Verification items for the finished model (mm, model axes). Face numbers are marked on the shaded views. A direction names the side the tool comes from. Give positions to 0.01 mm unless a question says otherwise; leave off trailing zeros. Order: outer loops, then holes, each group sorted by start corner. A loop starts at its lowest first (then second) coordinate and runs counter-clockwise, first axis right, second up. Notation, with made-up numbers: (1, 13) - (42, 13) arc R11 ccw to (42, 27) - close; hole circle Ø8 at (-17, 14). An arc over 180 degrees is marked (long way). Answer as a JSON object with one key per item and string values. Group by question number.
(1) Thickness scan on line 1 (Y direction, x = 20, z = 18); line 2 (X direction, y = -5, z = -10); line 3 (Z direction, x = -9.5, y = 11). Record the ranges inside material, lowest first.
(2) Section check B-B (x = 1). Record the boundary of the cut face in (y, z).
(3) Section check C-C (z = 12). Record the boundary of the cut face in (x, y), then the cut area to 3 significant figures.
(4) Section check D-D (x = -16.25). Record the boundary of the cut face in (y, z).
(5) Depth check by flat-ended pin: pin 1 Ø6.5 at (x, z) = (16.25, 12) entering from -Y; pin 2 Ø4 at (x, z) = (12.5, -2) entering from +Y; pin 3 Ø1.2 at (x, z) = (15.5, -10.5) entering from -Y; pin 4 Ø1 at (x, z) = (18, 11) entering from +Y. Enter the tip coordinate at first touch or a pass-through.
(6) Section check A-A (y = 17). Record the boundary of the cut face in (x, z).
(7) Access from +Z, -Z, +X, -X, +Y, -Y to the whole of each face (thin tool, end or side, straight path). Record for the marked faces 1, 2 and 3.
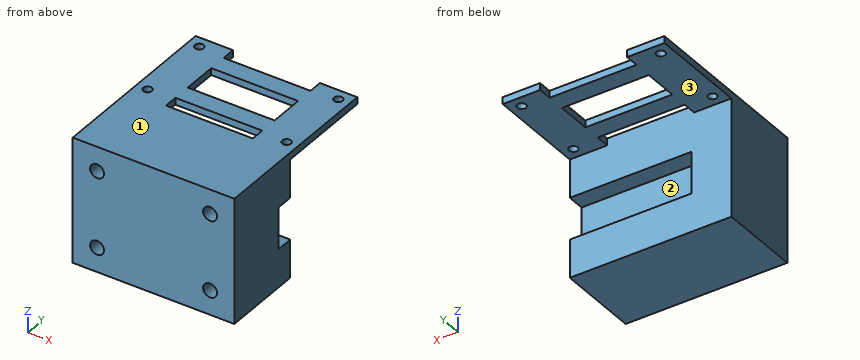
```python
from build123d import *

# Parameters (mm, degrees)
SKETCH1_W           = 46.5
SKETCH1_H           = 34
BOSS_EXTRUDE1_DEPTH = 13.75
SKETCH2_W           = 46.5
SKETCH2_H           = 42.25
BOSS_EXTRUDE2_DEPTH = 2
CUT_EXTRUDE1_REACH  = 62.18
SKETCH3_R           = 1.25
SKETCH3_W           = 25
SKETCH3_H           = 10
SKETCH4_W           = 35
SKETCH4_H           = 12
CUT_EXTRUDE2_DEPTH  = 5
SKETCH6_W           = 46.5
SKETCH6_H           = 36
SKETCH6_R           = 2
BOSS_EXTRUDE3_DEPTH = 10
SKETCH7_W           = 25
SKETCH7_H           = 4
CUT_EXTRUDE3_DEPTH  = 10


with BuildPart() as part:
    # Sketch1 → Boss-Extrude1 (new body)
    with BuildSketch(Plane(origin=(0, 0, 0), x_dir=(1, 0, 0), z_dir=(0, 1, 0))):
        Rectangle(SKETCH1_W, SKETCH1_H)
    extrude(amount=BOSS_EXTRUDE1_DEPTH)

    # Sketch2 → Boss-Extrude2 (add)
    with BuildSketch(Plane.XY.offset(17)):
        with Locations((0, 21.125)):
            Rectangle(SKETCH2_W, SKETCH2_H)
    extrude(amount=BOSS_EXTRUDE2_DEPTH)

    # Sketch3 → Cut-Extrude1 (cut, up to next)
    with BuildSketch(Plane.XY.offset(19), mode=Mode.PRIVATE) as cut_extrude1_sk1:
        with Locations((-20, 39)):
            Circle(SKETCH3_R)
    cut_extrude1_tool1 = extrude(cut_extrude1_sk1.sketch, amount=-CUT_EXTRUDE1_REACH, mode=Mode.PRIVATE) & part.part
    # Sketch3 → Cut-Extrude1 (cut, up to next)
    with BuildSketch(Plane.XY.offset(19), mode=Mode.PRIVATE) as cut_extrude1_sk2:
        with Locations(Location((20, 39, 0), (0, 0, 180))):
            Circle(SKETCH3_R)
    cut_extrude1_tool2 = extrude(cut_extrude1_sk2.sketch, amount=-CUT_EXTRUDE1_REACH, mode=Mode.PRIVATE) & part.part
    # Sketch3 → Cut-Extrude1 (cut, up to next)
    with BuildSketch(Plane.XY.offset(19), mode=Mode.PRIVATE) as cut_extrude1_sk3:
        with Locations((20, 17)):
            Circle(SKETCH3_R)
    cut_extrude1_tool3 = extrude(cut_extrude1_sk3.sketch, amount=-CUT_EXTRUDE1_REACH, mode=Mode.PRIVATE) & part.part
    # Sketch3 → Cut-Extrude1 (cut, up to next)
    with BuildSketch(Plane.XY.offset(19), mode=Mode.PRIVATE) as cut_extrude1_sk4:
        with Locations(Location((-20, 17, 0), (0, 0, 180))):
            Circle(SKETCH3_R)
    cut_extrude1_tool4 = extrude(cut_extrude1_sk4.sketch, amount=-CUT_EXTRUDE1_REACH, mode=Mode.PRIVATE) & part.part
    # Sketch3 → Cut-Extrude1 (cut, up to next)
    with BuildSketch(Plane.XY.offset(19), mode=Mode.PRIVATE) as cut_extrude1_sk5:
        with Locations((0, 28)):
            Rectangle(SKETCH3_W, SKETCH3_H)
    cut_extrude1_tool5 = extrude(cut_extrude1_sk5.sketch, amount=-CUT_EXTRUDE1_REACH, mode=Mode.PRIVATE) & part.part
    add(cut_extrude1_tool1.solids().sort_by_distance((-20, 39, 19))[0], mode=Mode.SUBTRACT)
    add(cut_extrude1_tool2.solids().sort_by_distance((20, 39, 19))[0], mode=Mode.SUBTRACT)
    add(cut_extrude1_tool3.solids().sort_by_distance((20, 17, 19))[0], mode=Mode.SUBTRACT)
    add(cut_extrude1_tool4.solids().sort_by_distance((-20, 17, 19))[0], mode=Mode.SUBTRACT)
    add(cut_extrude1_tool5.solids().sort_by_distance((0, 28, 19))[0], mode=Mode.SUBTRACT)

    # Sketch4 → Cut-Extrude2 (cut)
    with BuildSketch(Plane(origin=(0, 13.75, 0), x_dir=(1, 0, 0), z_dir=(0, 1, 0))):
        with Locations((5.75, 0)):
            Rectangle(SKETCH4_W, SKETCH4_H)
    extrude(amount=-CUT_EXTRUDE2_DEPTH, mode=Mode.SUBTRACT)

    # Sketch6 → Boss-Extrude3 (add)
    with BuildSketch(Plane.XZ):
        with Locations((0, 1)):
            Rectangle(SKETCH6_W, SKETCH6_H)
        with Locations(Location((16.25, -10, 0), (0, 0, 270))):
            Circle(SKETCH6_R, mode=Mode.SUBTRACT)
        with Locations(Location((-16.25, -10, 0), (0, 0, 270))):
            Circle(SKETCH6_R, mode=Mode.SUBTRACT)
        with Locations(Location((-16.25, 12, 0), (0, 0, 270))):
            Circle(SKETCH6_R, mode=Mode.SUBTRACT)
        with Locations(Location((16.25, 12, 0), (0, 0, 270))):
            Circle(SKETCH6_R, mode=Mode.SUBTRACT)
    extrude(amount=BOSS_EXTRUDE3_DEPTH)

    # Sketch7 → Cut-Extrude3 (cut)
    with BuildSketch(Plane(origin=(0, 0, 17), x_dir=(-1, 0, 0), z_dir=(0, 0, -1))):
        with Locations((0, 15.75)):
            Rectangle(SKETCH7_W, SKETCH7_H)
        with Locations((0, 40.25)):
            Rectangle(SKETCH7_W, SKETCH7_H)
    extrude(amount=-CUT_EXTRUDE3_DEPTH, mode=Mode.SUBTRACT)


solid = part.part
```
Solutions:
{
 "1": {"line 1": "y = -10 to 15.75, 18.25 to 37.75, 40.25 to 42.25", "line 2": "x = -23.25 to -18.25, -14.25 to 14.25, 18.25 to 23.25", "line 3": "z = -17 to -6, 6 to 19"},
 "2": {"outline": "(-10, -17) - (13.75, -17) - (13.75, -6) - (8.75, -6) - (8.75, 6) - (13.75, 6) - (13.75, 19) - (-10, 19) - close; (17.75, 17) - (23, 17) - (23, 19) - (17.75, 19) - close; (33, 17) - (38.25, 17) - (38.25, 19) - (33, 19) - close"},
 "3": {"outline": "(-23.25, -10) - (-18.25, -10) - (-18.25, 0) - (-14.25, 0) - (-14.25, -10) - (14.25, -10) - (14.25, 0) - (18.25, 0) - (18.25, -10) - (23.25, -10) - (23.25, 13.75) - (-23.25, 13.75) - close", "area": "1,020 mm2"},
 "4": {"outline": "(-10, -17) - (13.75, -17) - (13.75, 17) - (42.25, 17) - (42.25, 19) - (-10, 19) - (-10, 14) - (0, 14) - (0, 10) - (-10, 10) - (-10, -8) - (0, -8) - (0, -12) - (-10, -12) - close"},
 "5": {"pin 1": "stops at y = -10", "pin 2": "stops at y = 8.75", "pin 3": "stops at y = 0", "pin 4": "stops at y = 13.75"},
 "6": {"outline": "(-23.25, 17) - (-21.25, 17) - (-21.25, 19) - (-23.25, 19) - close; (-18.75, 17) - (-12.5, 17) - (-12.5, 19) - (-18.75, 19) - close; (12.5, 17) - (18.75, 17) - (18.75, 19) - (12.5, 19) - close; (21.25, 17) - (23.25, 17) - (23.25, 19) - (21.25, 19) - close"},
 "7": {"face 1": "+Z, +X, -X, +Y, -Y", "face 2": "+X, +Y", "face 3": "-Z, +X, -X, +Y"}
}
